```python
from build123d import *

# Parameters (mm, degrees)
HOLE1_D                      = 8
HOLE1_DEPTH                  = 10
F_5_16_CLEARANCE_HOLE1_D     = 8.376
F_5_16_CLEARANCE_HOLE1_DEPTH = 23
F_5_16_CLEARANCE_HOLE1_TIP   = 2.516404272
F_1_4_CLEARANCE_HOLE1_D      = 6.647
F_1_4_CLEARANCE_HOLE1_DEPTH  = 20
F_1_4_CLEARANCE_HOLE1_TIP    = 1.996960267
CHAMFER1_SIZE                = 0.5
CHAMFER6_SIZE                = 2
CHAMFER7_SIZE                = 2


with BuildPart() as part:
    # Sketch1 → Revolve1 (revolve)
    with BuildSketch(Plane(origin=(0, 0, 0), x_dir=(1, 0, 0), z_dir=(0, 1, 0))):
        Polygon((375, 4.500036707), (0, 4.500036707), (0, -320), (165, -320), (165, -263.511012034), (375, -15.499963293), align=None)
    revolve(axis=Axis((0, 0, -4.500036707), (0, 0, 1)))

    # Sketch2 → Cut-Revolve1 (revolve, cut)
    with BuildSketch(Plane(origin=(0, 0, 0), x_dir=(1, 0, 0), z_dir=(0, 1, 0))):
        Polygon((315, 4.500036707), (0, 4.500036707), (0, -320), (125, -320), (125, -270), (121, -270), (121, -255), (146, -255), (315, -55.410156014), align=None)
    revolve(axis=Axis((0, 0, -4.500036707), (0, 0, 1)), mode=Mode.SUBTRACT)

    # Hole1
    with Locations(Plane(origin=(0, 0, -4.500036707), x_dir=(-1, 0, 0), z_dir=(0, 0, -1))):
        with Locations((314.119041054, -130.112367004), (-314.119041054, 130.112367004)):
            Hole(HOLE1_D / 2, depth=HOLE1_DEPTH)

    # 5/16 Clearance Hole1
    with Locations(Plane(origin=(0, 0, -4.500036707), x_dir=(-1, 0, 0), z_dir=(0, 0, -1))):
        with Locations((0, -345), (-172.5, -298.778764306), (-298.778764306, -172.5), (-345, 0), (-298.778764306, 172.5), (-172.5, 298.778764306), (0, 345), (172.5, 298.778764306), (298.778764306, 172.5), (345, 0), (298.778764306, -172.5), (172.5, -298.778764306)):
            Hole(F_5_16_CLEARANCE_HOLE1_D / 2, depth=F_5_16_CLEARANCE_HOLE1_DEPTH)
            with Locations((0, 0, -(F_5_16_CLEARANCE_HOLE1_DEPTH + F_5_16_CLEARANCE_HOLE1_TIP / 2))):  # 118° drill point
                Cone(0, F_5_16_CLEARANCE_HOLE1_D / 2, F_5_16_CLEARANCE_HOLE1_TIP, mode=Mode.SUBTRACT)

    # 1/4 Clearance Hole1
    with Locations(Plane.XY.offset(320)):
        with Locations((-107.833784131, 107.833784131), (0, 152.5), (107.833784131, 107.833784131), (152.5, 0), (107.833784131, -107.833784131), (0, -152.5), (-107.833784131, -107.833784131), (-152.5, 0)):
            Hole(F_1_4_CLEARANCE_HOLE1_D / 2, depth=F_1_4_CLEARANCE_HOLE1_DEPTH)
            with Locations((0, 0, -(F_1_4_CLEARANCE_HOLE1_DEPTH + F_1_4_CLEARANCE_HOLE1_TIP / 2))):  # 118° drill point
                Cone(0, F_1_4_CLEARANCE_HOLE1_D / 2, F_1_4_CLEARANCE_HOLE1_TIP, mode=Mode.SUBTRACT)

    # Chamfer1
    chamfer1_edges = [part.edges().sort_by_distance(p)[0] for p in [
        (310.119041054, 130.112367004, -4.500036707),
        (-318.119041054, -130.112367004, -4.500036707),
        (-176.688, 298.778764306, -4.500036707),
        (-4.188, 345, -4.500036707),
        (168.312, 298.778764306, -4.500036707),
        (294.590764306, 172.5, -4.500036707),
        (340.812, 0, -4.500036707),
        (294.590764306, -172.5, -4.500036707),
        (168.312, -298.778764306, -4.500036707),
        (-4.188, -345, -4.500036707),
    ]]
    chamfer(chamfer1_edges, length=CHAMFER1_SIZE)

    # Chamfer6
    chamfer6_edges = [part.edges().sort_by_distance(p)[0] for p in [
        (-315, 0, -4.500036707),
    ]]
    chamfer(chamfer6_edges, length=CHAMFER6_SIZE)

    # Chamfer7
    chamfer7_edges = [part.edges().sort_by_distance(p)[0] for p in [
        (-165, 0, 320),
    ]]
    chamfer(chamfer7_edges, length=CHAMFER7_SIZE)


solid = part.part
```
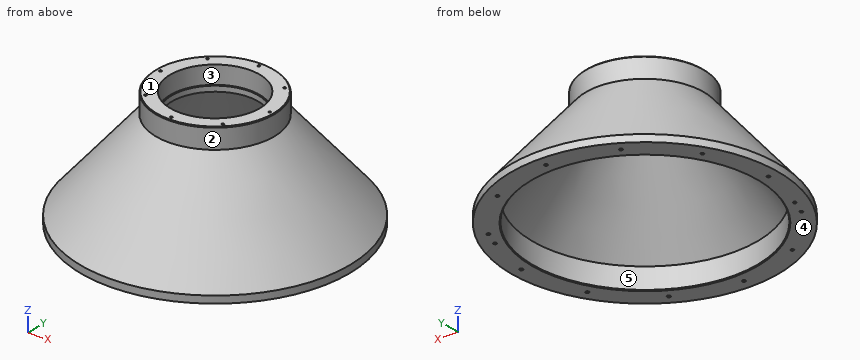
CAD build for the part. Positions are in the model's coordinates, mm. Face numbers are marked on the shaded views. A direction names the side the tool comes from. Coordinates: 2 decimals unless noted, no trailing zeros. Write each loop counter-clockwise with the first axis right and the second up, starting at its lowest first coordinate (ties: lowest second). Pieces come first, ordered by that corner, then holes. Notation, with made-up numbers: (-17.5, 41.5) -> (35.5, 41.5) arc R19 ccw to (35.5, 73.5) -> close; hole circle Ø9 at (-39, 18). An arc over 180 degrees is marked (long way). Return JSON: item names as keys, results as strings. Group by question number.
Q1. Pull direction Y, two halves, no side cores. Call the marked faces 1, 2 and 3: released by +Y, released by -Y, zero draft, split by the parting line, or undercut.
Q2. Drill centre lines: line 1 (X direction, y = 172.5, z = 8.5); line 2 (X direction, y = 19, z = 19.5); line 3 (Y direction, x = 47, z = 161). Where is each one in solid material? Low to high.
Q3. Which spindle directions (+Z, -Z, +X, -X, +Y, -Y) get a long thin tool onto all of the face, cutting with end or side? Do the marked faces 4 and 5. Say none if no direction does.
Q4. Cut at B-B, the plane z = 203.5. Give the cut face in (x, y).
Q5. Flat gauge pins, fed straight in: pin 1 (2 mm diameter, centred on y = -234.5, z = 44, fed in from +X); pin 2 (12 mm diameter, centred on y = 120, z = 141, fed in from +X); pin 3 (4 mm diameter, centred on x = 152.5, y = 0, fed in from -Z); pin 4 (9.5 mm diameter, centred on x = -298.78, y = 172.5, fed in from -Z). Where does each tip first touch, or does it go through?
Q6. Cut at A-A, the plane z = 289. Give the cut face in (x, y).
Returned:
{
 "1": {"face 1": "zero draft", "face 2": "split by the parting line", "face 3": "undercut"},
 "2": {"line 1": "x = -332.97 to -302.97, -294.59 to -263.57, 263.57 to 294.59, 302.97 to 332.97", "line 2": "x = -371.13 to -314.43, 314.43 to 371.13", "line 3": "y = -247.37 to -220.64, 220.64 to 247.37"},
 "3": {"face 4": "-Z, +X, -X, +Y, -Y", "face 5": "-Z"},
 "4": {"outline": "circle Ø431.63 at (0, 0); hole circle Ø379.21 at (0, 0)"},
 "5": {"pin 1": "stops at x = 262.44", "pin 2": "stops at x = 246.82", "pin 3": "stops at z = 244.96", "pin 4": "stops at z = -4.5"},
 "6": {"outline": "circle Ø330 at (0, 0); hole circle Ø250 at (0, 0)"}
}
